The figure shows three views and two pictorial views of one solid part (mm, origin at its lowest corner). Answer the questions. A direction names the side the tool comes from. Give positions to 0.01 mm unless a question says otherwise; leave off trailing zeros. Loops run counter-clockwise (first coordinate to the right, second up) from the corner with the lowest first, then second, coordinate; pieces in that order, holes last. Notation, with made-up numbers: M -40,20 L -2,20 A9 ccw -2,24 Z; hole C 20,70.5 d10. An arc over 180 degrees is marked long. Answer in a Markdown table with one row per item. Add a question column.
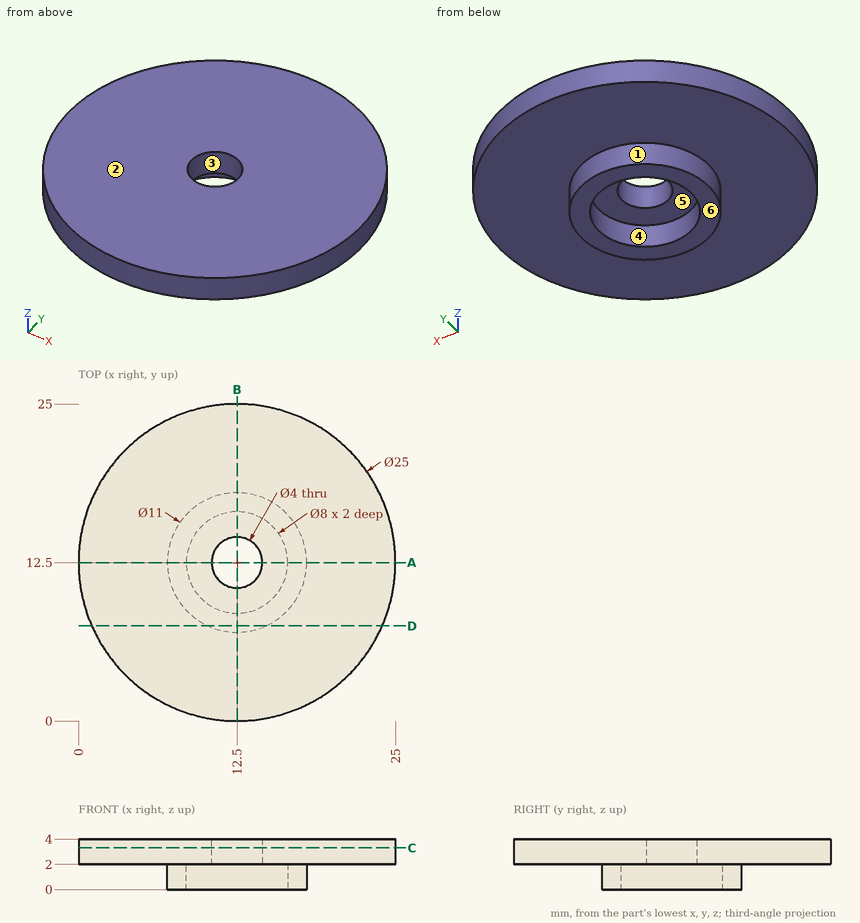
(1) Section C-C, the plane z = 3.3 is taken. Determine the outline of the cut face in (x, y).
(2) The mould has two halves that part along Y. Classify the marked faces 1, 2, 3 and 4: pulls with the +Y half, pulls with the -Y half, needs draft (parallel to the pull), parting line crosses it, or undercut.
(3) Section A-A, the plane y = 12.5 is taken. Determine the outline of the cut face in (x, z).
(4) Consider line 1 along Y through (x, z) = (12.5, 0.55); line 2 along Z through (x, y) = (4, 16); line 3 along X through (y, z) = (10.75, 0.45). Determine where each line is inside the solid, lowest interval first. Write a range as from..to.
(5) Section D-D, the plane y = 7.5 is taken. Determine the outline of the cut face in (x, z), and give its area (3 significant figures).
(6) Which of the six approach directions +Z, -Z, +X, -X, +Y, -Y give full straight-line access (tool end or side, diameter ignored) to the marked faces 5 and 6?
(7) Each of these flat-tipped pins is pushed along its axis until it touches: P1, Ø1, axis at y = 4.5, z = 2.5, coming from the +X side; P2, Ø1, axis at x = 9.5, z = 3.5, coming from the +Y side. Where does it stop, or does it pass through?
Numbers:
| question | item | result |
|---|---|---|
| 1 | outline | C 12.5,12.5 d25; hole C 12.5,12.5 d4 |
| 2 | face 1 | parting line crosses it |
| 2 | face 2 | needs draft |
| 2 | face 3 | undercut |
| 2 | face 4 | undercut |
| 3 | outline | M 0,2 L 7,2 L 7,0 L 8.5,0 L 8.5,2 L 10.5,2 L 10.5,4 L 0,4 Z; M 14.5,2 L 16.5,2 L 16.5,0 L 18,0 L 18,2 L 25,2 L 25,4 L 14.5,4 Z |
| 4 | line 1 | y = 7..8.5, 16.5..18 |
| 4 | line 2 | z = 2..4 |
| 4 | line 3 | x = 7.29..8.9, 16.1..17.71 |
| 5 | outline | M 1.04,2 L 10.21,2 L 10.21,0 L 14.79,0 L 14.79,2 L 23.96,2 L 23.96,4 L 1.04,4 Z |
| 5 | area | 55.0 mm² |
| 6 | face 5 | -Z |
| 6 | face 6 | -Z, +X, -X, +Y, -Y |
| 7 | P1 | stops at x = 22.5 |
| 7 | P2 | stops at y = 24.75 |
